Study the drawing (mm; zero at the part's minimum x, y, z) and answer. A direction names the side the tool comes from. Give positions to 0.01 mm unless a question says otherwise; leave off trailing zeros. Write each loop counter-clockwise with the first axis right and the second up, starting at its lowest first coordinate (ties: lowest second). Pieces come first, ordered by that corner, then holes. Notation, with made-up numbers: M 36.5,33.25 L 60.5,33.25 A10 ccw 60.5,37.25 Z; hole C -11,8.25 d5. An arc over 180 degrees is marked long. Use a Markdown table: item, result. Add a question column.
Item 1: Given P1, Ø10, axis at x = 47.5, y = 26.5, coming from the -Z side; P2, Ø5, axis at y = 50, z = 9.5, coming from the -X side; P3, Ø12, axis at x = 38, z = 16, coming from the +Y side; P4, Ø10, axis at x = 49.5, y = 18, coming from the +Z side, each flat-ended and moving along its own axis, determine where each tip first touches the part or whether it passes through.
Item 2: A cutting plane is placed at A-A on z = 7. Determine the outline of the cut face in (x, y) (1 decimal), then the cut area to 3 significant figures.
Item 3: A cutting plane is placed at D-D on z = 20. Determine the outline of the cut face in (x, y) (1 decimal).
Item 4: For the marked faces 4, 5 and 6, determine the directions among +Z, -Z, +X, -X, +Y, -Y from which every point of the face is accessible in a straight line to the end or side of a thin tool.
Item 5: The mould has two halves that part along X. Classify the marked faces 1, 2 and 3: pulls with the +X half, pulls with the -X half, needs draft (parallel to the pull), parting line crosses it, or undercut.
Item 6: A cutting plane is placed at B-B on y = 26.5. Determine the outline of the cut face in (x, z) (1 decimal), then the cut area to 3 significant figures.
Item 7: A cutting plane is placed at C-C on x = 34.5. Determine the outline of the cut face in (y, z), then the cut area to 3 significant figures.
Item 8: Consider probe 1 along X at (y, z) = (45.5, 9.25) (1 decimal); probe 2 along X at (y, z) = (31.5, 18.5) (1 decimal); probe 3 along Z at (x, y) = (74, 7). Determine where each line is inside the solid, lowest interval first. Write a range as [from, to].
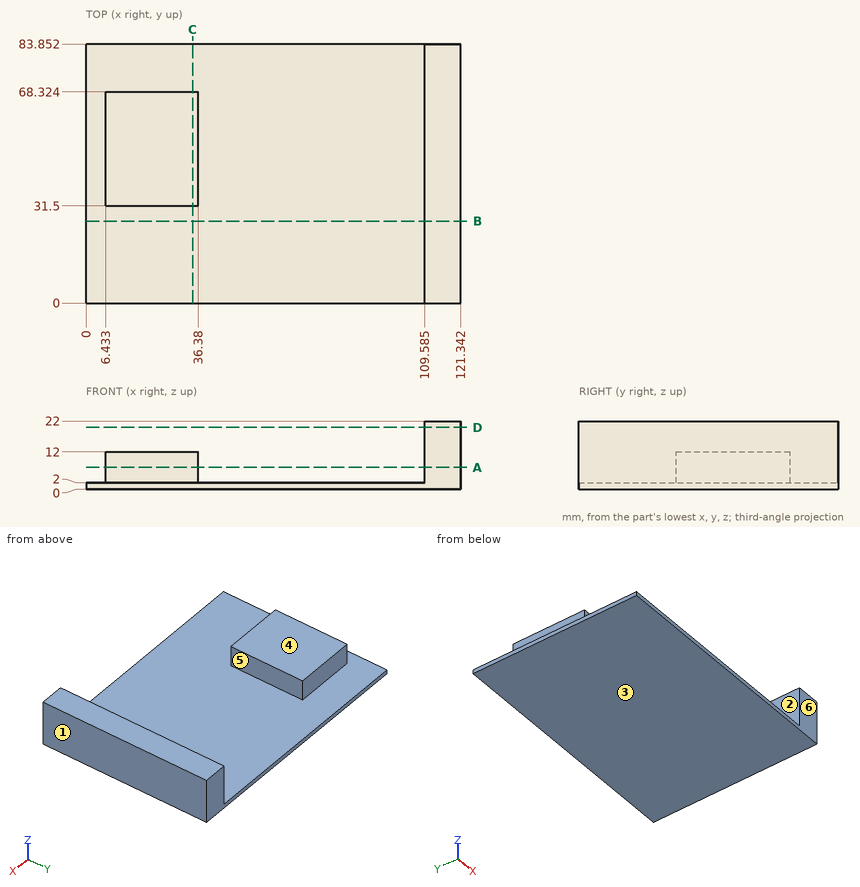
Filled in:
| question | item | result |
|---|---|---|
| 1 | P1 | z = 0 |
| 1 | P2 | x = 6.43 |
| 1 | P3 | y = 68.32 |
| 1 | P4 | z = 2 |
| 2 | outline | M 6.4,31.5 L 36.4,31.5 L 36.4,68.3 L 6.4,68.3 Z; M 109.6,0 L 121.3,0 L 121.3,83.9 L 109.6,83.9 Z |
| 2 | area | 2,090 mm² |
| 3 | outline | M 109.6,0 L 121.3,0 L 121.3,83.9 L 109.6,83.9 Z |
| 4 | face 4 | +Z, -X, +Y, -Y |
| 4 | face 5 | +Z, +Y, -Y |
| 4 | face 6 | +Z, -Z, +X, -X, -Y |
| 5 | face 1 | pulls with the +X half |
| 5 | face 2 | undercut |
| 5 | face 3 | needs draft |
| 6 | outline | M 0,0 L 121.3,0 L 121.3,22 L 109.6,22 L 109.6,2 L 0,2 Z |
| 6 | area | 478 mm² |
| 7 | outline | M 0,0 L 83.85,0 L 83.85,2 L 68.32,2 L 68.32,12 L 31.5,12 L 31.5,2 L 0,2 Z |
| 7 | area | 536 mm² |
| 8 | probe 1 | [6.4, 36.4], [109.6, 121.3] |
| 8 | probe 2 | [109.6, 121.3] |
| 8 | probe 3 | [0, 2] |
